Autodesk Fusion 360 part; units mm, degrees
sketch "Esboço1" plane through (0, 0, 0) normal (0, 0, 1) x (1, 0, 0)
  line L0 (0, 5) -> (0, 6.96) construction
  line L1 (-4.9294, -0.8373) -> (-10.6041, 32.5691)
  line L2 (4.9294, -0.8373) -> (10.6041, 32.5691)
  arc A0 (10.6041, 32.5691) -> (-10.6041, 32.5691) centre (0, 21.96) ccw
  arc A1 (-4.9294, -0.8373) -> (4.9294, -0.8373) centre (0, 0) ccw
  circle A2 centre (0, 0) radius 3
  circle A3 centre (0, 0) radius 1.65
  dimension "d1" = 10
  dimension "d2" = 21.96
  dimension "d3" = 30
  dimension "d4" = 33.885
  dimension "d5" = 33.885
  dimension "d8" = 6
  dimension "d9" = 3.3
extrude "Extrusão1" add sketch "Esboço1" along normal blind 5 contours L1 L2 A0 A1 | A2 | A3
extrude "Extrusão2" cut sketch "Esboço1" along normal blind 28 contours A3
extrude "Extrusão3" cut sketch "Esboço1" along normal blind 3.75 contours A2
chamfer "Chanfro1" distance 2 angle 45 2 edges at (7.7667, 15.8659, 5) (-7.7667, 15.8659, 5)
chamfer "Chanfro2" distance 4 angle 45 1 edges at (0, 36.96, 5)
Geometry check sheet. Reference: the model listing, model coordinates, mm. A direction names the side the tool comes from. Give positions to 0.01 mm unless a question says otherwise; leave off trailing zeros. Loops run counter-clockwise (first coordinate to the right, second up) from the corner with the lowest first, then second, coordinate; pieces in that order, holes last. Notation, with made-up numbers: M 43,81.5 L 56,81.5 A34 cw 56,113.5 Z; hole C 17,63.25 d3. An arc over 180 degrees is marked long. Write item = value, one per line.
(1) Material ranges on line 1 (Y direction, x = 0, z = 4.65); line 2 (Y direction, x = 0, z = 4.4); line 3 (X direction, y = 32.5, z = 2.8), recorded low to high. Write a range as [from, to].
Answer below:
line_1 = [-3.35, -1.65], [1.65, 33.31]
line_2 = [-3.6, -1.65], [1.65, 33.56]
line_3 = [-7.95, 7.95]
(2) Release check for a two-part mould opening along X. For faces 1 (the face through (-0.15, 34.1, 3.86)), 2 (the face through (-1.216, -1.115, 4.366)), 3 (the face through (-6.54, 14.56, 3.99)), 4 (the face through (7.727, 15.632, 1.479)) record: released by +X, released by -X, zero draft, split by the parting line, or undercut.
Answer below:
face_1 = split by the parting line
face_2 = undercut
face_3 = released by -X
face_4 = released by +X
(3) Sectioned sample at A-A, the plane x = 0. Record the cut outline in (y, z), plus the area to 3 significant figures.
Answer below:
outline = M -5,0 L -3,0 L -3,3.75 L -1.65,3.75 L -1.65,5 L -3,5 L -5,3 Z; M 1.65,3.75 L 3,3.75 L 3,0 L 36.96,0 L 36.96,1 L 32.96,5 L 1.65,5 Z
area = 173 mm2
(4) Sectioned sample at C-C, the plane z = 4.2. Record the cut outline in (x, y), plus the area to 3 significant figures.
Answer below:
outline = M -8.9,29.71 L -3.75,-0.64 A3.8 ccw 3.75,-0.64 L 8.9,29.71 A11.8 ccw Z; hole C 0,0 d3.3
area = 443 mm2
(5) Tool access check on faces 5 (the face through (0, -5, 1)), 6 (the face through (1.3, -1.3, 3.75)). Record the directions out of +Z, -Z, +X, -X, +Y, -Y that give a thin tool (end or side, any length) a straight path to the whole face; none if there is none.
Answer below:
face_5 = +Z, -Z, -Y
face_6 = -Z
(6) Gauge pin test, flat ends, axial feed: pin 1 Ø2 at (x, y) = (-1, -0.5) entering from -Z; pin 2 Ø1 at (y, z) = (8.5, 2.5) entering from +X. Record the tip position at first contact, or that the pin passes through.
Answer below:
pin_1 = 3.75
pin_2 = 6.6
(7) Sectioned sample at B-B, the plane y = 0. Record the cut outline in (x, z).
Answer below:
outline = M -5.07,0 L -3,0 L -3,3.75 L -1.65,3.75 L -1.65,5 L -3.04,5 L -5.07,3 Z; M 1.65,3.75 L 3,3.75 L 3,0 L 5.07,0 L 5.07,3 L 3.04,5 L 1.65,5 Z
